from build123d import *

# Parameters (mm, degrees)
F0_W     = 260
F0_H     = 50
F1_DEPTH = 5
F2_W     = 20
F2_H     = 50
F3_DEPTH = 45
F4_R     = 6
F5_DEPTH = 5


with BuildPart() as f1:
    # F0 (on Front) → F1 (new body)
    with BuildSketch(Plane.XZ):
        with Locations((7.377451, -32.76636)):
            Rectangle(F0_W, F0_H)
    extrude(amount=F1_DEPTH)

    # F2 (on face) → F3 (join)
    with BuildSketch(Plane(origin=(0, 0, 0), x_dir=(-1, 0, 0), z_dir=(0, 1, 0))):
        with Locations((-17.377451, -32.76636)):
            Rectangle(F2_W, F2_H)
    extrude(amount=F3_DEPTH)

    # F4 (on Front) → F5 (cut, through all)
    with BuildSketch(Plane.XZ):
        with Locations((122.377451, -42.76636)):
            Circle(F4_R)
        with Locations((122.377451, -22.76636)):
            Circle(F4_R)
        with Locations((-107.622549, -42.76636)):
            Circle(F4_R)
        with Locations((-107.622549, -22.76636)):
            Circle(F4_R)
    extrude(amount=F5_DEPTH, mode=Mode.SUBTRACT)


solid = f1.part
For this review, take the finished solid that the model builds, in its own axes (mm). A direction names the side the tool comes from. Coordinates: 2 decimals unless noted, no trailing zeros. Order: outer loops, then holes, each group sorted by start corner. A loop starts at its lowest first (then second) coordinate and runs counter-clockwise, first axis right, second up. Notation, with made-up numbers: (43.25, 72) - (90.25, 72) arc R19 ccw to (90.25, 100) - close; hole circle Ø2 at (-11.75, 55.5). An arc over 180 degrees is marked (long way). Answer as CSV lines item,"result". Start each with the question number.
1) Add section D-D (y = 30). State the section outline as (x, z) points.
2) Insertion check: P1, Ø4, axis at y = 31.5, z = -48.5, coming from the -X side; P2, Ø1.5, axis at x = -66, z = -22.5, coming from the +Y side; P3, Ø4, axis at x = 41.5, y = 1.5, coming from the -Z side; P4, Ø22.5, axis at y = 15.5, z = -33, coming from the +X side. Each pin has a flat end and moves straight along its axis. Give the tip position at first contact, or say it passes through.
3) Add section A-A (z = -32). State the section outline as (x, y) points, then the cut area to 3 significant figures.
4) Draft analysis for pull direction Z (two halves, no side actions). For faces 4 (the flat face through (27.377, 22, -33)), 5 (the cylindrical face through (121.077, -2.465, -28.624)), 6 (the flat face through (16, 7, -7.766)), state which applies: +Z half, -Z half, draft (parallel to the pull), parting line (faces both ways), or undercut.
5) Add section C-C (z = -20). State the section outline as (x, y) points.
6) To check wall thickness, follow line 1 along Y through (x, z) = (-93.5, -23); line 2 along X through (y, z) = (3, -38.5). State the ranges of each line that lie inside material, in increasing order. Write a range as [from, to].
7) Add section B-B (x = -14). State the section outline as (y, z) points.
8) Machinability: for faces 1 (the flat face through (18, 45, -32)), 2 (the flat face through (-59, 0, -32)), 3 (the flat face through (82, 0, -32)), which of the approach directions +Z, -Z, +X, -X, +Y, -Y give a long, thin tool a straight path to every point of the face, cutting with its end or side? Answer none if there is none.
Result:
1,outline,"(7.38, -57.77) - (27.38, -57.77) - (27.38, -7.77) - (7.38, -7.77) - close"
2,P1,"x = 7.38"
2,P2,"y = 0"
2,P3,"z = -57.77"
2,P4,"x = 27.38"
3,outline,"(-122.62, -5) - (137.38, -5) - (137.38, 0) - (27.38, 0) - (27.38, 45) - (7.38, 45) - (7.38, 0) - (-122.62, 0) - close"
3,area,"2,200 mm^2"
4,face 4,"draft"
4,face 5,"undercut"
4,face 6,"+Z half"
5,outline,"(-122.62, -5) - (-112.95, -5) - (-112.95, 0) - (-122.62, 0) - close; (-102.3, -5) - (117.05, -5) - (117.05, 0) - (27.38, 0) - (27.38, 45) - (7.38, 45) - (7.38, 0) - (-102.3, 0) - close; (127.7, -5) - (137.38, -5) - (137.38, 0) - (127.7, 0) - close"
6,line 1,"[-5, 0]"
6,line 2,"[7.38, 27.38]"
7,outline,"(-5, -57.77) - (0, -57.77) - (0, -7.77) - (-5, -7.77) - close"
8,face 1,"+Z, -Z, +X, -X, +Y"
8,face 2,"+Z, -Z, -X, +Y"
8,face 3,"+Z, -Z, +X, +Y"
